from build123d import *

# Parameters (mm, degrees)
SKETCH_3_W           = 89.2
SKETCH_3_H           = 95.8
SKETCH_3_R           = 1.65
EXTRUDE_1_DEPTH      = 3
EXTRUDE_1_DEPTH_BACK = 0.0001
SKETCH_6_W           = 3
SKETCH_6_H           = 95.8
EXTRUDE_3_DEPTH      = 42.8
SKETCH_8_R           = 1.1
CUT_EXTRUDE_6_DEPTH  = 47.8
SKETCH_8_9_R         = 1.1
CUT_EXTRUDE_7_DEPTH  = 47.8
SKETCH_8_10_R        = 1.1
CUT_EXTRUDE_8_DEPTH  = 47.8
SKETCH_8_11_R        = 1.1
CUT_EXTRUDE_9_DEPTH  = 47.8
SKETCH_12_R          = 2.5
CUT_EXTRUDE_10_DEPTH = 47.8
SKETCH_12_4_R        = 2.5
CUT_EXTRUDE_11_DEPTH = 47.8
CUT_EXTRUDE_21_DEPTH = 19.978934005
SKETCH_16_W          = 3
SKETCH_16_H          = 16.067623689
EXTRUDE_4_DEPTH      = 3
SKETCH_17_W          = 16.067623689
SKETCH_17_H          = 3
CUT_EXTRUDE_22_DEPTH = 3
CUT_EXTRUDE_23_DEPTH = 10
FILLET_1_R           = 3
FILLET_2_R           = 3
FILLET_3_R           = 3
FILLET_4_R           = 3


with BuildPart() as part:
    # Sketch 3 → Extrude 1 (new body, two sides)
    with BuildSketch(Plane(origin=(0, 0, 0), x_dir=(1, 0, 0), z_dir=(0, 1, 0))) as extrude_1_sk:
        with Locations((44.6, -47.9)):
            Rectangle(SKETCH_3_W, SKETCH_3_H)
        with Locations(Location((18, -23.4, 0), (0, 0, 270))):  # turned: the seam where the file's is
            Circle(SKETCH_3_R, mode=Mode.SUBTRACT)
        with Locations(Location((71.2, -23.4, 0), (0, 0, 270))):  # turned: the seam where the file's is
            Circle(SKETCH_3_R, mode=Mode.SUBTRACT)
        with Locations(Location((18, -72.4, 0), (0, 0, 270))):  # turned: the seam where the file's is
            Circle(SKETCH_3_R, mode=Mode.SUBTRACT)
        with Locations(Location((71.2, -72.4, 0), (0, 0, 270))):  # turned: the seam where the file's is
            Circle(SKETCH_3_R, mode=Mode.SUBTRACT)
        with Locations(Location((6, -19.15, 0), (0, 0, 270))):  # turned: the seam where the file's is
            Circle(SKETCH_3_R, mode=Mode.SUBTRACT)
        with Locations(Location((54.8, -19.15, 0), (0, 0, 270))):  # turned: the seam where the file's is
            Circle(SKETCH_3_R, mode=Mode.SUBTRACT)
        with Locations(Location((6, -76.65, 0), (0, 0, 270))):  # turned: the seam where the file's is
            Circle(SKETCH_3_R, mode=Mode.SUBTRACT)
        with Locations(Location((54.8, -76.65, 0), (0, 0, 270))):  # turned: the seam where the file's is
            Circle(SKETCH_3_R, mode=Mode.SUBTRACT)
    extrude(amount=EXTRUDE_1_DEPTH)
    extrude(extrude_1_sk.sketch, amount=-EXTRUDE_1_DEPTH_BACK)

    # Sketch 6 → Extrude 3 (add)
    with BuildSketch(Plane.XZ.offset(0.0001)):
        with Locations((-1.5, 47.9)):
            Rectangle(SKETCH_6_W, SKETCH_6_H)
    extrude(amount=-EXTRUDE_3_DEPTH)

    # Sketch 8 → Cut-Extrude 6 (cut)
    with BuildSketch(Plane.ZY.offset(3)):
        with Locations((86.6, 37.8)):
            Circle(SKETCH_8_R)
    extrude(amount=-CUT_EXTRUDE_6_DEPTH, mode=Mode.SUBTRACT)

    # Sketch 8_9 → Cut-Extrude 7 (cut)
    with BuildSketch(Plane.ZY.offset(3)):
        with Locations((9.2, 37.8)):
            Circle(SKETCH_8_9_R)
    extrude(amount=-CUT_EXTRUDE_7_DEPTH, mode=Mode.SUBTRACT)

    # Sketch 8_10 → Cut-Extrude 8 (cut)
    with BuildSketch(Plane.ZY.offset(3)):
        with Locations((9.2, 20)):
            Circle(SKETCH_8_10_R)
    extrude(amount=-CUT_EXTRUDE_8_DEPTH, mode=Mode.SUBTRACT)

    # Sketch 8_11 → Cut-Extrude 9 (cut)
    with BuildSketch(Plane.ZY.offset(3)):
        with Locations((86.6, 20)):
            Circle(SKETCH_8_11_R)
    extrude(amount=-CUT_EXTRUDE_9_DEPTH, mode=Mode.SUBTRACT)

    # Sketch 12 → Cut-Extrude 10 (cut)
    with BuildSketch(Plane.ZY.offset(3)):
        with Locations((18.2, 37.8)):
            Circle(SKETCH_12_R)
    extrude(amount=-CUT_EXTRUDE_10_DEPTH, mode=Mode.SUBTRACT)

    # Sketch 12_4 → Cut-Extrude 11 (cut)
    with BuildSketch(Plane.ZY.offset(3)):
        with Locations((77.6, 37.8)):
            Circle(SKETCH_12_4_R)
        with Locations((77.6, 20)):
            Circle(SKETCH_12_4_R)
        with Locations((18.2, 37.8)):
            Circle(SKETCH_12_4_R)
        with Locations((18.2, 20)):
            Circle(SKETCH_12_4_R)
    extrude(amount=-CUT_EXTRUDE_11_DEPTH, mode=Mode.SUBTRACT)

    # Sketch 13 → Cut-Extrude 21 (cut)
    with BuildSketch(Plane.XZ.offset(0.0001)):
        Polygon((-5, 47.9), (-5, 57.401139719), (0, 57.401139719), (0, 41.33351603), (-5, 41.33351603), align=None)
    extrude(amount=-CUT_EXTRUDE_21_DEPTH, mode=Mode.SUBTRACT)

    # Sketch 16 → Extrude 4 (add)
    with BuildSketch(Plane.XZ.offset(0.0001)):
        with Locations((-1.5, 49.367327875)):
            Rectangle(SKETCH_16_W, SKETCH_16_H)
    extrude(amount=-EXTRUDE_4_DEPTH)

    # Sketch 17 → Cut-Extrude 22 (cut)
    with BuildSketch(Plane.ZY.offset(3)):
        with Locations((49.367327875, 1.4999)):
            Rectangle(SKETCH_17_W, SKETCH_17_H)
    extrude(amount=-CUT_EXTRUDE_22_DEPTH, mode=Mode.SUBTRACT)

    # Sketch 18 → Cut-Extrude 23 (cut)
    with BuildSketch(Plane.ZY.offset(3)):
        with BuildLine():
            Line((19.009554581, 2.875833037), (15.037851313, 2.875833037))
            ThreePointArc((15.037851313, 2.875833037), (13.91378435, 3.9999), (15.037851313, 5.123966963))
            Line((15.037851313, 5.123966963), (19.009554581, 5.123966963))
            ThreePointArc((19.009554581, 5.123966963), (20.133621543, 3.9999), (19.009554581, 2.875833037))
        make_face()
        with BuildLine():
            Line((15.037851313, 12.123966963), (19.009554581, 12.123966963))
            ThreePointArc((19.009554581, 12.123966963), (20.133621543, 10.9999), (19.009554581, 9.875833037))
            Line((19.009554581, 9.875833037), (15.037851313, 9.875833037))
            ThreePointArc((15.037851313, 9.875833037), (13.91378435, 10.9999), (15.037851313, 12.123966963))
        make_face()
    extrude(amount=-CUT_EXTRUDE_23_DEPTH, mode=Mode.SUBTRACT)

    # Fillet 1
    fillet_1_edges = [part.edges().sort_by_distance(p)[0] for p in [
        (-1.5, 42.7999, 95.8),
    ]]
    fillet(fillet_1_edges, radius=FILLET_1_R)

    # Fillet 2
    fillet_2_edges = [part.edges().sort_by_distance(p)[0] for p in [
        (-1.5, 42.7999, 0),
    ]]
    fillet(fillet_2_edges, radius=FILLET_2_R)

    # Fillet 3
    fillet_3_edges = [part.edges().sort_by_distance(p)[0] for p in [
        (89.2, 1.49995, 95.8),
    ]]
    fillet(fillet_3_edges, radius=FILLET_3_R)

    # Fillet 4
    fillet_4_edges = [part.edges().sort_by_distance(p)[0] for p in [
        (89.2, 1.49995, 0),
    ]]
    fillet(fillet_4_edges, radius=FILLET_4_R)


solid = part.part
Work out the finished part from the listing and answer in its coordinate system (mm). A direction names the side the tool comes from. Round coordinates to 2 decimals unless told otherwise and drop trailing zeros. Loops run counter-clockwise (first coordinate to the right, second up) from the corner with the lowest first, then second, coordinate; pieces in that order, holes last. Notation, with made-up numbers: M 55.5,44.25 L 72.5,44.25 A16 cw 72.5,59.25 Z; hole C 76.5,46 d9. An arc over 180 degrees is marked long. One line per question, with ' | ' between items. Start each with the question number.
(1) A cutting plane is placed at D-D on z = 76.65. Write down the section's boundary in (x, y).
(2) A cutting plane is placed at A-A on y = 13.5. Write down the section's boundary in (x, z).
(3) A tool of negligible diameter and unlimited length cuts with its end or side. For faces 5 (the face through (0, 2, 49)), 6 (the face through (-2, 9.876, 17)), 7 (the face through (44, 3, 47)), 8 (the face through (-1, 19.979, 49)), 9 (the face through (2, 2.876, 17)), from which of +Z, -Z, +X, -X, +Y, -Y can it reach the whole face along a straight path? Write none if from no direction.
(4) A cutting plane is placed at B-B on x = 54.8. Write down the section's boundary in (y, z), plus the area to 3 significant figures.
(5) For a pull along Y with two mould halves and no side action, classify faces 1 (the face through (-2, 5.124, 17)), 2 (the face through (-1.521, 36.726, 8.962)), 3 (the face through (-1.48, 41.94, 0.9)), 4 (the face through (89.2, 2, 49)) as released by +Y, released by -Y, zero draft, split by the parting line, or undercut.
(6) A cutting plane is placed at C-C on z = 23.4. Write down the section's boundary in (x, y).
(7) Flat-ended cylindrical pins translate along their axes: pin 1 Ø4 at (y, z) = (20, 18.2) entering from -X; pin 2 Ø5.5 at (x, z) = (18, 23.4) entering from +Y; pin 3 Ø3 at (y, z) = (31.5, 19) entering from +X. Find the tip coordinate at first contact, or state that the pin passes through.
(8) Find the intervals of material crossed by line 1 (Y direction, x = -1.85, z = 18.2); line 2 (Y direction, x = 55.5, z = 37); line 3 (X direction, y = 19, z = 8), in increasing order.
Geometry check:
1) outline: M -3,0 L 4.35,0 L 4.35,3 L 0,3 L 0,17.69 L -3,17.69 Z; M -3,22.31 L 0,22.31 L 0,35.49 L -3,35.49 Z; M -3,40.11 L 0,40.11 L 0,42.8 L -3,42.8 Z; M 7.65,0 L 53.15,0 L 53.15,3 L 7.65,3 Z; M 56.45,0 L 89.2,0 L 89.2,3 L 56.45,3 Z
2) outline: M -3,0 L 0,0 L 0,41.33 L -3,41.33 Z; M -3,57.4 L 0,57.4 L 0,95.8 L -3,95.8 Z
3) face 5: -X, -Y | face 6: +X, -X | face 7: +Z, -Z, +X, +Y | face 8: +X, -X, -Y | face 9: -X
4) outline: M 0,0 L 3,0 L 3,17.5 L 0,17.5 Z; M 0,20.8 L 3,20.8 L 3,75 L 0,75 Z; M 0,78.3 L 3,78.3 L 3,95.8 L 0,95.8 Z | area: 268 mm²
5) face 1: undercut | face 2: undercut | face 3: released by +Y | face 4: zero draft
6) outline: M -3,0 L 16.35,0 L 16.35,3 L 0,3 L 0,42.8 L -3,42.8 Z; M 19.65,0 L 69.55,0 L 69.55,3 L 19.65,3 Z; M 72.85,0 L 89.2,0 L 89.2,3 L 72.85,3 Z
7) pin 1: passes through | pin 2: stops at y = 3 | pin 3: stops at x = 0
8) line 1: y = 0 to 2.88, 5.12 to 9.88, 12.12 to 17.5, 22.5 to 35.3, 40.3 to 42.8 | line 2: y = 0 to 3 | line 3: x = -3 to 0
